Input: part model. Units: mm. Frame: model coordinates. Give positions to 0.01 mm unless a question says otherwise; leave off trailing zeros. Order: outer loops, then holes, each group sorted by start corner. A loop starts at its lowest first (then second) coordinate and runs counter-clockwise, first axis right, second up. Notation, with made-up numbers: M 32.5,23 L 74.5,23 A16 cw 74.5,46 Z; hole C -1.5,8.5 d9. An arc over 180 degrees is marked long. Use a Markdown table: item, result.
Autodesk Inventor part; units mm, degrees
ref_plane "YZ Plane" through (0, 0, 0) normal (1, 0, 0) x (0, 1, 0)
ref_plane "XZ Plane" through (0, 0, 0) normal (0, 1, 0) x (-1, 0, 0)
ref_plane "XY Plane" through (0, 0, 0) normal (0, 0, 1) x (1, 0, 0)
sketch "Sketch1" plane through (0, 0, 0) normal (1, 0, 0) x (0, 1, 0)
  circle A0 centre (0, 0) radius 44
  dimension "d0" = 88
extrude "Extrusion1" add sketch "Sketch1" along normal blind 10
sketch "Sketch2" plane through (10, 0, 0) normal (1, 0, 0) x (0, 0, -1)
  circle A0 centre (0, 0) radius 7.5
  dimension "d3" = 15
extrude "Extrusion2" cut sketch "Sketch2" against normal through all
sketch "Sketch3" plane through (10, 0, 0) normal (1, 0, 0) x (0, 0, -1)
  circle A0 centre (-22, -20) radius 7.5
  point P0 (0, 0)
  dimension "d6" = 15
extrude "Extrusion3" cut sketch "Sketch3" against normal through all
properties part number "disk"
1) Cut plane C-C on x = 8.75. Return loops of the section in (y, z).
Response values:
| item | result |
|---|---|
| outline | C 0,0 d88; hole C -20,22 d15; hole C 0,0 d15 |
2) First-contact query: pin 1 Ø4 at (x, z) = (2, -16.5) entering from +Y; pin 2 Ø4 at (x, y) = (5, -17) entering from -Z; pin 3 Ø6 at (x, z) = (4, -17.5) entering from -Y. Flat tips, straight axial feed; report the tip coordinate or a pass-through.
Response values:
| item | result |
|---|---|
| pin 1 | stops at y = 41.54 |
| pin 2 | stops at z = -41.36 |
| pin 3 | stops at y = -41.54 |
3) Mould query, pull axis Z, two halves, no side actions, for faces 1 (the face through (4.93, -9.538, 42.954)), 2 (the face through (0, -1, -9)), 3 (the face through (5.07, -19.67, 29.493)). Classes: released by +Z, released by -Z, zero draft, split by the parting line, or undercut.
Response values:
| item | result |
|---|---|
| face 1 | split by the parting line |
| face 2 | zero draft |
| face 3 | undercut |
4) Cut plane A-A on z = 0. Return loops of the section in (x, y).
Response values:
| item | result |
|---|---|
| outline | M 0,-44 L 10,-44 L 10,-7.5 L 0,-7.5 Z; M 0,7.5 L 10,7.5 L 10,44 L 0,44 Z |
5) Cut plane D-D on z = 33. Return loops of the section in (x, y), and give its area (3 significant figures).
Response values:
| item | result |
|---|---|
| outline | M 0,-29.1 L 10,-29.1 L 10,29.1 L 0,29.1 Z |
| area | 582 mm² |
6) Material intervals for line 1 (Y direction, x = 2.75, z = 22); line 2 (Y direction, x = 2.75, z = 1.5); line 3 (Y direction, x = 1.75, z = -37.5), sorted ascending. Write a range as from..to.
Response values:
| item | result |
|---|---|
| line 1 | y = -38.11..-27.5, -12.5..38.11 |
| line 2 | y = -43.97..-7.35, 7.35..43.97 |
| line 3 | y = -23.02..23.02 |
